from build123d import *

# Parameters (mm, degrees)
SKETCH1_W           = 92
SKETCH1_H           = 120
BOSS_EXTRUDE1_DEPTH = 8
SKETCH2_W           = 9.4
SKETCH2_H           = 120
BOSS_EXTRUDE2_DEPTH = 72
CUT_EXTRUDE1_REACH  = 173.067
SKETCH3_R           = 3
SKETCH3_R_2         = 1.5
CUT_EXTRUDE2_REACH  = 173.067
SKETCH4_R           = 1.25
SKETCH5_R           = 2.5
CUT_EXTRUDE3_DEPTH  = 172.067238243


with BuildPart() as part:
    # Sketch1 → Boss-Extrude1 (new body)
    with BuildSketch(Plane(origin=(0, 0, 0), x_dir=(1, 0, 0), z_dir=(0, 1, 0))):
        with Locations((46, 60)):
            Rectangle(SKETCH1_W, SKETCH1_H)
    extrude(amount=BOSS_EXTRUDE1_DEPTH)

    # Sketch2 → Boss-Extrude2 (add)
    with BuildSketch(Plane(origin=(0, 8, 0), x_dir=(1, 0, 0), z_dir=(0, 1, 0))):
        with Locations((4.7, 60)):
            Rectangle(SKETCH2_W, SKETCH2_H)
        with Locations((87.3, 60)):
            Rectangle(SKETCH2_W, SKETCH2_H)
    extrude(amount=BOSS_EXTRUDE2_DEPTH)

    # Sketch3 → Cut-Extrude1 (cut, up to next)
    with BuildSketch(Plane.XZ, mode=Mode.PRIVATE) as cut_extrude1_sk1:
        with Locations(Location((31.4, -92.5, 0), (0, 0, 270))):
            Circle(SKETCH3_R)
    cut_extrude1_tool1 = extrude(cut_extrude1_sk1.sketch, amount=-CUT_EXTRUDE1_REACH, mode=Mode.PRIVATE) & part.part
    # Sketch3 → Cut-Extrude1 (cut, up to next)
    with BuildSketch(Plane.XZ, mode=Mode.PRIVATE) as cut_extrude1_sk2:
        with Locations(Location((31.4, -110, 0), (0, 0, 270))):
            Circle(SKETCH3_R_2)
    cut_extrude1_tool2 = extrude(cut_extrude1_sk2.sketch, amount=-CUT_EXTRUDE1_REACH, mode=Mode.PRIVATE) & part.part
    # Sketch3 → Cut-Extrude1 (cut, up to next)
    with BuildSketch(Plane.XZ, mode=Mode.PRIVATE) as cut_extrude1_sk3:
        with Locations(Location((31.4, -10, 0), (0, 0, 270))):
            Circle(SKETCH3_R_2)
    cut_extrude1_tool3 = extrude(cut_extrude1_sk3.sketch, amount=-CUT_EXTRUDE1_REACH, mode=Mode.PRIVATE) & part.part
    # Sketch3 → Cut-Extrude1 (cut, up to next)
    with BuildSketch(Plane.XZ, mode=Mode.PRIVATE) as cut_extrude1_sk4:
        with Locations(Location((31.4, -27.5, 0), (0, 0, 270))):
            Circle(SKETCH3_R)
    cut_extrude1_tool4 = extrude(cut_extrude1_sk4.sketch, amount=-CUT_EXTRUDE1_REACH, mode=Mode.PRIVATE) & part.part
    add(cut_extrude1_tool1.solids().sort_by_distance((31.4, 0, -92.5))[0], mode=Mode.SUBTRACT)
    add(cut_extrude1_tool2.solids().sort_by_distance((31.4, 0, -110))[0], mode=Mode.SUBTRACT)
    add(cut_extrude1_tool3.solids().sort_by_distance((31.4, 0, -10))[0], mode=Mode.SUBTRACT)
    add(cut_extrude1_tool4.solids().sort_by_distance((31.4, 0, -27.5))[0], mode=Mode.SUBTRACT)

    # Sketch4 → Cut-Extrude2 (cut, up to next)
    with BuildSketch(Plane(origin=(92, 0, 0), x_dir=(0, 0, -1), z_dir=(1, 0, 0)), mode=Mode.PRIVATE) as cut_extrude2_sk1:
        with Locations((5.5, 44.5)):
            Circle(SKETCH4_R)
    cut_extrude2_tool1 = extrude(cut_extrude2_sk1.sketch, amount=-CUT_EXTRUDE2_REACH, mode=Mode.PRIVATE) & part.part
    # Sketch4 → Cut-Extrude2 (cut, up to next)
    with BuildSketch(Plane(origin=(92, 0, 0), x_dir=(0, 0, -1), z_dir=(1, 0, 0)), mode=Mode.PRIVATE) as cut_extrude2_sk2:
        with Locations((36.5, 44.5)):
            Circle(SKETCH4_R)
    cut_extrude2_tool2 = extrude(cut_extrude2_sk2.sketch, amount=-CUT_EXTRUDE2_REACH, mode=Mode.PRIVATE) & part.part
    # Sketch4 → Cut-Extrude2 (cut, up to next)
    with BuildSketch(Plane(origin=(92, 0, 0), x_dir=(0, 0, -1), z_dir=(1, 0, 0)), mode=Mode.PRIVATE) as cut_extrude2_sk3:
        with Locations((5.5, 13.5)):
            Circle(SKETCH4_R)
    cut_extrude2_tool3 = extrude(cut_extrude2_sk3.sketch, amount=-CUT_EXTRUDE2_REACH, mode=Mode.PRIVATE) & part.part
    # Sketch4 → Cut-Extrude2 (cut, up to next)
    with BuildSketch(Plane(origin=(92, 0, 0), x_dir=(0, 0, -1), z_dir=(1, 0, 0)), mode=Mode.PRIVATE) as cut_extrude2_sk4:
        with Locations((36.5, 13.5)):
            Circle(SKETCH4_R)
    cut_extrude2_tool4 = extrude(cut_extrude2_sk4.sketch, amount=-CUT_EXTRUDE2_REACH, mode=Mode.PRIVATE) & part.part
    # Sketch4 → Cut-Extrude2 (cut, up to next)
    with BuildSketch(Plane(origin=(92, 0, 0), x_dir=(0, 0, -1), z_dir=(1, 0, 0)), mode=Mode.PRIVATE) as cut_extrude2_sk5:
        with Locations((83.5, 13.5)):
            Circle(SKETCH4_R)
    cut_extrude2_tool5 = extrude(cut_extrude2_sk5.sketch, amount=-CUT_EXTRUDE2_REACH, mode=Mode.PRIVATE) & part.part
    # Sketch4 → Cut-Extrude2 (cut, up to next)
    with BuildSketch(Plane(origin=(92, 0, 0), x_dir=(0, 0, -1), z_dir=(1, 0, 0)), mode=Mode.PRIVATE) as cut_extrude2_sk6:
        with Locations((114.5, 13.5)):
            Circle(SKETCH4_R)
    cut_extrude2_tool6 = extrude(cut_extrude2_sk6.sketch, amount=-CUT_EXTRUDE2_REACH, mode=Mode.PRIVATE) & part.part
    # Sketch4 → Cut-Extrude2 (cut, up to next)
    with BuildSketch(Plane(origin=(92, 0, 0), x_dir=(0, 0, -1), z_dir=(1, 0, 0)), mode=Mode.PRIVATE) as cut_extrude2_sk7:
        with Locations((83.5, 44.5)):
            Circle(SKETCH4_R)
    cut_extrude2_tool7 = extrude(cut_extrude2_sk7.sketch, amount=-CUT_EXTRUDE2_REACH, mode=Mode.PRIVATE) & part.part
    # Sketch4 → Cut-Extrude2 (cut, up to next)
    with BuildSketch(Plane(origin=(92, 0, 0), x_dir=(0, 0, -1), z_dir=(1, 0, 0)), mode=Mode.PRIVATE) as cut_extrude2_sk8:
        with Locations((114.5, 44.5)):
            Circle(SKETCH4_R)
    cut_extrude2_tool8 = extrude(cut_extrude2_sk8.sketch, amount=-CUT_EXTRUDE2_REACH, mode=Mode.PRIVATE) & part.part
    add(cut_extrude2_tool1.solids().sort_by_distance((92, 44.5, -5.5))[0], mode=Mode.SUBTRACT)
    add(cut_extrude2_tool2.solids().sort_by_distance((92, 44.5, -36.5))[0], mode=Mode.SUBTRACT)
    add(cut_extrude2_tool3.solids().sort_by_distance((92, 13.5, -5.5))[0], mode=Mode.SUBTRACT)
    add(cut_extrude2_tool4.solids().sort_by_distance((92, 13.5, -36.5))[0], mode=Mode.SUBTRACT)
    add(cut_extrude2_tool5.solids().sort_by_distance((92, 13.5, -83.5))[0], mode=Mode.SUBTRACT)
    add(cut_extrude2_tool6.solids().sort_by_distance((92, 13.5, -114.5))[0], mode=Mode.SUBTRACT)
    add(cut_extrude2_tool7.solids().sort_by_distance((92, 44.5, -83.5))[0], mode=Mode.SUBTRACT)
    add(cut_extrude2_tool8.solids().sort_by_distance((92, 44.5, -114.5))[0], mode=Mode.SUBTRACT)

    # Sketch5 → Cut-Extrude3 (cut, through all)
    with BuildSketch(Plane(origin=(92, 0, 0), x_dir=(0, 0, -1), z_dir=(1, 0, 0))):
        with Locations((18, 71)):
            Circle(SKETCH5_R)
        with Locations((102, 71)):
            Circle(SKETCH5_R)
    extrude(amount=-CUT_EXTRUDE3_DEPTH, mode=Mode.SUBTRACT)


solid = part.part
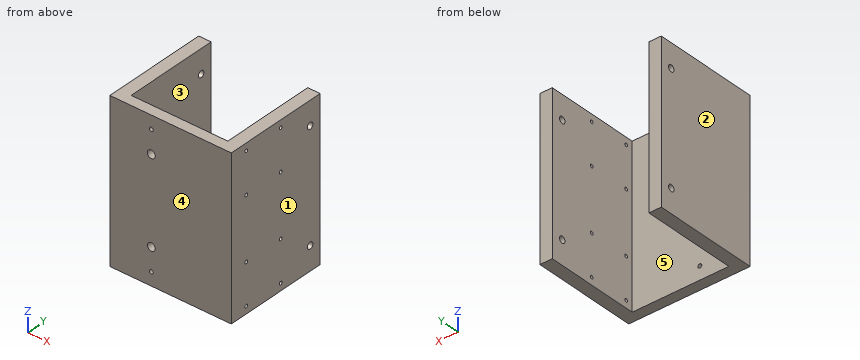
Here's how the part is built. I have some questions about the finished solid (model axes, mm). Face numbers are marked on the shaded views. A direction names the side the tool comes from. Give positions to 0.01 mm unless a question says otherwise; leave off trailing zeros. Order: outer loops, then holes, each group sorted by start corner. A loop starts at its lowest first (then second) coordinate and runs counter-clockwise, first axis right, second up. Notation, with made-up numbers: M 52,20 L 84,20 A35 cw 84,56 Z; hole C 42,31.5 d3. An arc over 180 degrees is marked long. Answer as a JSON object with one key per item and string values. Group by question number.
1) Suppose I cut it at D-D, the plane z = -68.5. Write out the boundary of the cut face in (x, y).
2) We'd pull the mould along X, two halves only. Please class the marked faces 1, 2 and 3: pulls with the +X half, pulls with the -X half, needs draft (parallel to the pull), parting line crosses it, or undercut.
3) On a 3-axis mill with a long thin cutter (end or side, diameter ignored), from which of +Z, -Z, +X, -X, +Y, -Y can I reach the whole of each face in a straight line? I mean the marked faces 4 and 5. Say none if no direction works.
4) Suppose I cut it at A-A, the plane z = -10. Write out the boundary of the cut face in (x, y), plus the area to 3 significant figures.
5) Suppose I cut it at C-C, the plane z = -27.5. Write out the boundary of the cut face in (x, y).
6) Suppose I cut it at B-B, the plane y = 66. Write out the boundary of the cut face in (x, z).
7) Please list where these lines run through material, in increasing order: L1, parallel to Y at x = 90.25, z = -83.5; L2, parallel to X at y = 20, z = -48.5; L3, parallel to Y at x = 88, z = -83. Write a range as [from, to].
8) I'm going to push flat-ended pins straight in: pin 1 Ø2 at (y, z) = (44.5, -36.5) entering from +X; pin 2 Ø4 at (x, z) = (19, -48) entering from +Y. Where does each tip first touch, or does it pass through?
Results found:
{
 "1": {"outline": "M 0,0 L 92,0 L 92,80 L 82.6,80 L 82.6,8 L 9.4,8 L 9.4,80 L 0,80 Z"},
 "2": {"face 1": "pulls with the +X half", "face 2": "pulls with the -X half", "face 3": "undercut"},
 "3": {"face 4": "+Z, -Z, +X, -X, -Y", "face 5": "+Z, -Z, +Y"},
 "4": {"outline": "M 0,0 L 29.9,0 L 29.9,8 L 9.4,8 L 9.4,80 L 0,80 Z; M 32.9,0 L 92,0 L 92,80 L 82.6,80 L 82.6,8 L 32.9,8 Z", "area": "2,070 mm²"},
 "5": {"outline": "M 0,0 L 28.4,0 L 28.4,8 L 9.4,8 L 9.4,80 L 0,80 Z; M 34.4,0 L 92,0 L 92,80 L 82.6,80 L 82.6,8 L 34.4,8 Z"},
 "6": {"outline": "M 0,-120 L 9.4,-120 L 9.4,0 L 0,0 Z; M 82.6,-120 L 92,-120 L 92,0 L 82.6,0 Z"},
 "7": {"L1": "[0, 12.25], [14.75, 43.25], [45.75, 80]", "L2": "[0, 9.4], [82.6, 92]", "L3": "[0, 12.35], [14.65, 43.35], [45.65, 80]"},
 "8": {"pin 1": "x = 9.4", "pin 2": "y = 8"}
}
